from build123d import *

# Parameters (mm, degrees)
SKETCH1_W            = 15.8
SKETCH1_H            = 3.2
BOSS_EXTRUDE1_DEPTH  = 15.8
SKETCH2_R            = 2.4
BOSS_EXTRUDE2_DEPTH  = 1.6
SKETCH10_R           = 1.7
CUT_EXTRUDE8_DEPTH   = 1.6
LPATTERN1_COUNT      = 2
LPATTERN1_PITCH      = 8
LPATTERN1_COUNT_DIR2 = 2
LPATTERN1_PITCH_DIR2 = 8
SKETCH3_W            = 13.4
SKETCH3_H            = 13.4
CUT_EXTRUDE1_DEPTH   = 3
BOSS_EXTRUDE3_DEPTH  = 6.9
SKETCH8_R            = 2.9
CUT_EXTRUDE6_DEPTH   = 1.2
CUT_EXTRUDE7_START   = -5.7
SKETCH9_R            = 2.3
CUT_EXTRUDE7_DEPTH   = 28.741778513


with BuildPart() as part:
    # Sketch1 → Boss-Extrude1 (new body)
    with BuildSketch(Plane.XY):
        with Locations((7.9, 1.6)):
            Rectangle(SKETCH1_W, SKETCH1_H)
    extrude(amount=-BOSS_EXTRUDE1_DEPTH)

    # Sketch2 → Boss-Extrude2 (add)
    with BuildSketch(Plane(origin=(0, 3.2, 0), x_dir=(1, 0, 0), z_dir=(0, 1, 0))):
        with Locations(Location((3.9, 3.9, 0), (0, 0, 270))):
            Circle(SKETCH2_R)
    boss_extrude2 = extrude(amount=BOSS_EXTRUDE2_DEPTH)

    # Sketch10 → Cut-Extrude8 (cut)
    with BuildSketch(Plane(origin=(0, 4.8, 0), x_dir=(1, 0, 0), z_dir=(0, 1, 0))):
        with Locations(Location((3.9, 3.9, 0), (0, 0, 270))):
            Circle(SKETCH10_R)
    cut_extrude8 = extrude(amount=-CUT_EXTRUDE8_DEPTH, mode=Mode.SUBTRACT)

    # LPattern1: Boss-Extrude2, Cut-Extrude8 2 × 2
    with Locations(*[(j * LPATTERN1_PITCH_DIR2, 0, -i * LPATTERN1_PITCH) for i in range(LPATTERN1_COUNT) for j in range(LPATTERN1_COUNT_DIR2) if (i, j) != (0, 0)]):
        add(boss_extrude2)
        add(cut_extrude8, mode=Mode.SUBTRACT)

    # Sketch3 → Cut-Extrude1 (cut)
    with BuildSketch(Plane.XZ):
        with Locations((7.9, -7.9)):
            Rectangle(SKETCH3_W, SKETCH3_H)
    extrude(amount=-CUT_EXTRUDE1_DEPTH, mode=Mode.SUBTRACT)

    # Sketch4 → Boss-Extrude3 (add)
    with BuildSketch(Plane.XY):
        with BuildLine():
            Line((11.9, 0), (11.9, 3.2))
            Line((11.9, 3.2), (3.9, 3.2))
            Line((3.9, 3.2), (3.9, 0))
            ThreePointArc((3.9, 0), (7.9, -4), (11.9, 0))
        make_face()
    boss_extrude3 = extrude(amount=-BOSS_EXTRUDE3_DEPTH)

    # Sketch8 → Cut-Extrude6 (cut)
    with BuildSketch(Plane.XY):
        with Locations((7.9, 0)):
            Circle(SKETCH8_R)
    cut_extrude6 = extrude(amount=-CUT_EXTRUDE6_DEPTH, mode=Mode.SUBTRACT)

    # Sketch9 → Cut-Extrude7 (cut)
    with BuildSketch(Plane.XY.offset(-1.2).offset(CUT_EXTRUDE7_START)):
        with Locations((7.9, 0)):
            Circle(SKETCH9_R)
    cut_extrude7 = extrude(amount=CUT_EXTRUDE7_DEPTH, mode=Mode.SUBTRACT)

    # Mirror1: Boss-Extrude3, Cut-Extrude6, Cut-Extrude7 across plane
    add(boss_extrude3.mirror(Plane.XY.offset(-7.9)))
    add(cut_extrude6.mirror(Plane.XY.offset(-7.9)), mode=Mode.SUBTRACT)
    add(cut_extrude7.mirror(Plane.XY.offset(-7.9)), mode=Mode.SUBTRACT)


solid = part.part
Source: CAD feature listing. Evaluate the final solid. Frame: model axes, mm. A direction names the side the tool comes from. Round coordinates to 2 decimals unless told otherwise and drop trailing zeros. Loops run counter-clockwise (first coordinate to the right, second up) from the corner with the lowest first, then second, coordinate; pieces in that order, holes last.
Q1. Mould query, pull axis X, two halves, no side actions, for faces 5 (the face through (3.9, 2, -12)), 6 (the face through (4, 4.8, -6)), 7 (the face through (0, 2, -8)). Classes: pulls with the +X half, pulls with the -X half, needs draft (parallel to the pull), parting line crosses it, or undercut.
Q2. Section D-D, the plane y = -0.25. Return loops of the section in (x, z), plus the area to 3 significant figures.
Q3. Ray query, line 1 (X direction, y = 2.5, z = -1.25); line 2 (X direction, y = 3.75, z = -12); line 3 (Z direction, x = 11.9, y = 3.7). Return the intervals inside material, ascending.
Q4. Section B-B, the plane x = 7.9. Return loops of the section in (y, z).
Q5. Section A-A, the plane y = 3.5. Return loops of the section in (x, z).
Q6. Access query for faces 1 (the face through (1, 0, -8)), 2 (the face through (12, 3.2, -12)), 3 (the face through (6.075, -1.4, -4.09)), 4 (the face through (11.9, 1, -4)). Directions: +Z, -Z, +X, -X, +Y, -Y. A direction counts if a zero-diameter tool reaches every point of the face in a straight line with its end or side. Return the directions, or none.
Q7. Section C-C, the plane z = -9.25. Return loops of the section in (x, y), plus the area to 3 significant figures.
Q8. First-contact query: P1, Ø1.7, axis at x = 3, z = -3.5, coming from the +Y side; P2, Ø3, axis at x = 4.5, z = -9, coming from the -Y side; P3, Ø1, axis at y = -1, z = -2, coming from the -X side; P4, Ø3, axis at x = 2, z = -10.5, coming from the -Y side. Flat tips, straight axial feed; report the tip coordinate or a pass-through.
Solutions:
1. face 5: undercut
1. face 6: needs draft
1. face 7: pulls with the -X half
2. outline: (3.91, -15.8) - (5.01, -15.8) - (5.01, -14.6) - (5.61, -14.6) - (5.61, -8.9) - (3.91, -8.9) - close; (3.91, -6.9) - (5.61, -6.9) - (5.61, -1.2) - (5.01, -1.2) - (5.01, 0) - (3.91, 0) - close; (10.19, -14.6) - (10.79, -14.6) - (10.79, -15.8) - (11.89, -15.8) - (11.89, -8.9) - (10.19, -8.9) - close; (10.19, -6.9) - (11.89, -6.9) - (11.89, 0) - (10.79, 0) - (10.79, -1.2) - (10.19, -1.2) - close
2. area: 44.2 mm2
3. line 1: x = 0 to 1.2, 3.9 to 11.9, 14.6 to 15.8
3. line 2: x = 1.5 to 2.2, 5.6 to 6.3, 9.5 to 10.2, 13.6 to 14.3
3. line 3: z = -14.3 to -13.6, -10.2 to -9.5, -6.3 to -5.6, -2.2 to -1.5
4. outline: (-4, -15.8) - (-2.9, -15.8) - (-2.9, -14.6) - (-2.3, -14.6) - (-2.3, -8.9) - (-4, -8.9) - close; (-4, -6.9) - (-2.3, -6.9) - (-2.3, -1.2) - (-2.9, -1.2) - (-2.9, 0) - (-4, 0) - close; (2.3, -14.6) - (2.9, -14.6) - (2.9, -15.8) - (3.2, -15.8) - (3.2, 0) - (2.9, 0) - (2.9, -1.2) - (2.3, -1.2) - (2.3, -6.9) - (3, -6.9) - (3, -8.9) - (2.3, -8.9) - close
5. outline: circle Ø4.8 at (3.9, -11.9); circle Ø4.8 at (3.9, -3.9); circle Ø4.8 at (11.9, -11.9); circle Ø4.8 at (11.9, -3.9); hole circle Ø3.4 at (3.9, -11.9); hole circle Ø3.4 at (3.9, -3.9); hole circle Ø3.4 at (11.9, -11.9); hole circle Ø3.4 at (11.9, -3.9)
6. face 1: +Z, -Z, -X, -Y
6. face 2: +Y
6. face 3: +Z, -Z
6. face 4: -Y
7. outline: (0, 0) - (1.2, 0) - (1.2, 3) - (3.9, 3) - (3.9, 0) arc R4 ccw to (11.9, 0) - (11.9, 3) - (14.6, 3) - (14.6, 0) - (15.8, 0) - (15.8, 3.2) - (0, 3.2) - close; hole circle Ø4.6 at (7.9, 0)
7. area: 42.9 mm2
8. P1: stops at y = 4.8
8. P2: stops at y = -3.52
8. P3: stops at x = 3.93
8. P4: stops at y = 0
